CAD build for the part. Positions are in the model's coordinates, mm. Coordinates: 2 decimals unless noted, no trailing zeros. Loops run counter-clockwise (first coordinate to the right, second up) from the corner with the lowest first, then second, coordinate; pieces in that order, holes last. Notation, with made-up numbers: M 28,40.25 L 49,40.25 A12 ccw 49,51.25 Z; hole C 15,7.25 d7. An arc over 180 degrees is marked long. Answer as a JSON object with one key per item and string values. Group by question number.
```python
from build123d import *

# Parameters (mm, degrees)
SKETCH_1_W          = 50
SKETCH_1_H          = 60
EXTRUDE_1_DEPTH     = 3
SKETCH_2_W          = 10
SKETCH_2_H          = 3
EXTRUDE_2_DEPTH     = 3
CUT_EXTRUDE_1_DEPTH = 42.509035161
SKETCH_4_R          = 7.05
CUT_EXTRUDE_2_DEPTH = 42.509035161
SKETCH_5_R          = 1.6
SKETCH_5_W          = 3.2
SKETCH_5_H          = 10.1
CUT_EXTRUDE_3_DEPTH = 42.509035161
SKETCH_7_R          = 0.75
CUT_EXTRUDE_4_DEPTH = 42.509035161
FILLET_1_R          = 10


with BuildPart() as part:
    # 草图1 → 凸台-拉伸1 (new body)
    with BuildSketch(Plane(origin=(0, 0, 0), x_dir=(1, 0, 0), z_dir=(0, 1, 0))):
        Rectangle(SKETCH_1_W, SKETCH_1_H)
    extrude(amount=EXTRUDE_1_DEPTH)

    # 草图2 → 凸台-拉伸2 (add)
    with BuildSketch(Plane(origin=(0, 3, 0), x_dir=(1, 0, 0), z_dir=(0, 1, 0))):
        with Locations((-10, -31.5)):
            Rectangle(SKETCH_2_W, SKETCH_2_H)
        with Locations((10, -31.5)):
            Rectangle(SKETCH_2_W, SKETCH_2_H)
    extrude(amount=-EXTRUDE_2_DEPTH)

    # 草图3 → 切除-拉伸1 (cut, through all)
    with BuildSketch(Plane(origin=(0, 3, 0), x_dir=(1, 0, 0), z_dir=(0, 1, 0))):
        Polygon((-1.55, -30), (-1.55, -26), (-3, -26), (-3, -21), (-1.55, -21), (-1.55, -16), (1.55, -16), (1.55, -21), (3, -21), (3, -26), (1.55, -26), (1.55, -30), align=None)
    extrude(amount=-CUT_EXTRUDE_1_DEPTH, mode=Mode.SUBTRACT)

    # 草图4 → 切除-拉伸2 (cut, through all)
    with BuildSketch(Plane(origin=(0, 3, 0), x_dir=(1, 0, 0), z_dir=(0, 1, 0))):
        with Locations(Location((0, 7.290233074, 0), (0, 0, 270))):
            Circle(SKETCH_4_R)
    extrude(amount=-CUT_EXTRUDE_2_DEPTH, mode=Mode.SUBTRACT)

    # 草图5 → 切除-拉伸3 (cut, through all)
    with BuildSketch(Plane.XZ):
        with Locations(Location((13.5, 25, 0), (0, 0, 270))):
            Circle(SKETCH_5_R)
        with Locations(Location((-13.5, 25, 0), (0, 0, 90))):
            Circle(SKETCH_5_R)
        with Locations((20, 10)):
            Rectangle(SKETCH_5_W, SKETCH_5_H)
        with Locations((-20, 10)):
            Rectangle(SKETCH_5_W, SKETCH_5_H)
    extrude(amount=-CUT_EXTRUDE_3_DEPTH, mode=Mode.SUBTRACT)

    # 草图7 → 切除-拉伸4 (cut, through all)
    with BuildSketch(Plane.XZ):
        with Locations((-21.6, 15.05)):
            Circle(SKETCH_7_R)
        with Locations((-18.4, 15.05)):
            Circle(SKETCH_7_R)
        with Locations((-18.4, 4.95)):
            Circle(SKETCH_7_R)
        with Locations((-21.6, 4.95)):
            Circle(SKETCH_7_R)
        with Locations((21.6, 4.95)):
            Circle(SKETCH_7_R)
        with Locations((18.4, 4.95)):
            Circle(SKETCH_7_R)
        with Locations((18.4, 15.05)):
            Circle(SKETCH_7_R)
        with Locations((21.6, 15.05)):
            Circle(SKETCH_7_R)
        with Locations((-15, 30)):
            Circle(SKETCH_7_R)
        with Locations((-5, 30)):
            Circle(SKETCH_7_R)
        with Locations((5, 30)):
            Circle(SKETCH_7_R)
        with Locations((15, 30)):
            Circle(SKETCH_7_R)
    extrude(amount=-CUT_EXTRUDE_4_DEPTH, mode=Mode.SUBTRACT)

    # 圆角1
    fillet_1_edges = [part.edges().sort_by_distance(p)[0] for p in [
        (-25, 1.5, -30),
        (25, 1.5, -30),
    ]]
    fillet(fillet_1_edges, radius=FILLET_1_R)


solid = part.part
```
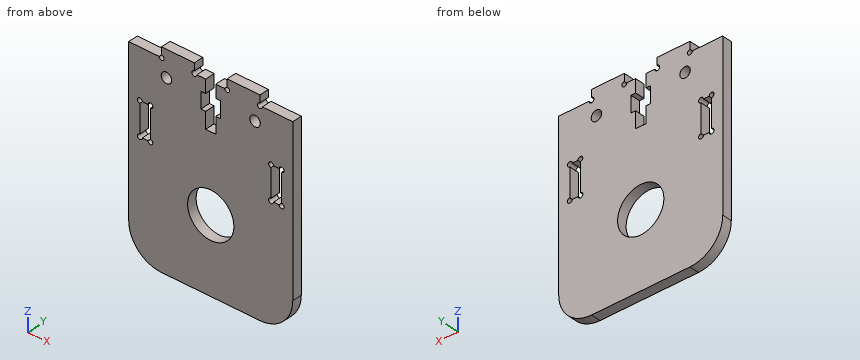
Item 1: Slice it at C-C, the plane z = -23. Write the cut outline in (x, y), then the cut area to 3 significant figures.
Item 2: Drill centre lines: L1, parallel to X at y = 2.2, z = 25; L2, parallel to X at y = 1.6, z = 27; L3, parallel to Z at x = -18, y = 1.8. Where is each one in solid material? Low to high. Write a range as from..to.
Item 3: Pin check, flat tips, straight feed: pin 1 (1.5 mm diameter, centred on x = -21.5, y = 1, fed in from +Z); pin 2 (1.1 mm diameter, centred on y = 2, z = 32, fed in from -X). Stop position of each tip, or through.
Item 4: Slice it at A-A, the plane z = -6. Write the cut outline in (x, y).
Item 5: Slice it at B-B, the plane y = 0.8. Count the separate pieces of the cut face and the enclosed holes in it, then the cut area to 3 significant figures.
Computed:
{
 "1": {"outline": "M -24.54,0 L 24.54,0 L 24.54,3 L -24.54,3 Z", "area": "147 mm2"},
 "2": {"L1": "-25..-15.1, -11.9..-3, 3..11.9, 15.1..25", "L2": "-25..-1.55, 1.55..25", "L3": "-29.54..4.32, 5.58..14.42, 15.68..30"},
 "3": {"pin 1": "z = 30", "pin 2": "x = -15"},
 "4": {"outline": "M -25,0 L -6.93,0 L -6.93,3 L -25,3 Z; M 6.93,0 L 25,0 L 25,3 L 6.93,3 Z"},
 "5": {"separate pieces": "1", "enclosed holes": "5", "area": "2,710 mm2"}
}
